Verification items for the finished model (mm, model axes). Face numbers are marked on the shaded views. Round coordinates to 2 decimals unless told otherwise and drop trailing zeros. Order: outer loops, then holes, each group sorted by start corner. A loop starts at its lowest first (then second) coordinate and runs counter-clockwise, first axis right, second up. Notation, with made-up numbers: M 47.25,3.25 L 65.25,3.25 A19 cw 65.25,17.25 Z; hole C 67,89.25 d5. An arc over 180 degrees is marked long. Use CSV: the item, a comma, the result in double quotes. Start each with the question number.
Q1. Scan lines: line 1 (Y direction, x = -77, z = 3.75) (1 decimal); line 2 (X direction, y = 24, z = 4.25); line 3 (Z direction, x = -8, y = -4). Record each from-to range of solid material in increasing order.
Q2. Sectioned sample at A-A (z = 2.75). Enter the section's corners in (x, y), and give its area (3 significant figures).
Q3. Sectioned sample at D-D (x = -106). Enter the section's corners in (y, z), and give its area (3 significant figures).
Q4. Gauge pin test, flat ends, axial feed: pin 1 Ø5 at (x, y) = (-81.5, -31.5) entering from -Z; pin 2 Ø6.5 at (x, y) = (80, 26) entering from -Z; pin 3 Ø1 at (y, z) = (25, 0) entering from -X; pin 4 Ø1.7 at (y, z) = (-24, -2) entering from -X. Record the tip position at first contact, or that the pin passes through.
Q5. Sectioned sample at B-B (y = -12.5). Enter the section's corners in (x, z).
Q6. Sectioned sample at C-C (x = 53). Enter the section's corners in (y, z).
Q7. Mould release check, pull along X, two halves, no side actions. Record for the marked faces 1, 2, 3 and 4: +X half, -X half, draft (parallel to the pull), parting line (faces both ways), or undercut.
```python
from build123d import *

# Parameters (mm, degrees)
F2_DEPTH  = 3
F3_DEPTH  = 7.9
F4_DEPTH  = 7.9
F5_DEPTH  = 3
F6_R      = 5
F6_2_R    = 5
F9_D      = 3
F10_DEPTH = 4
F11_DEPTH = 4


with BuildPart() as f2:
    # F0 (on Top) → F2 (new body)
    with BuildSketch(Plane.XY):
        with BuildLine():
            ThreePointArc((68.6448413014, 3.4252903424), (74.3230858808, 21.4851908555), (83.8, 37.8739237785))
            Line((83.8, 37.8739237785), (-65.6162592679, 37.8739237785))
            ThreePointArc((-65.6162592679, 37.8739237785), (-82.3199649398, 11.4193737584), (-82.519158721, -19.8666825891))
            Line((-82.519158721, -19.8666825891), (-73.9695476283, -37.2867286205))
            Line((-73.9695476283, -37.2867286205), (83.8, -37.2867286205))
            ThreePointArc((83.8, -37.2867286205), (75.2631412951, -21.4263167299), (69.0877699379, -4.5060504646))
            ThreePointArc((69.0877699379, -4.5060504646), (68.3487291916, -0.5692843065), (68.6448413014, 3.4252903424))
        make_face()
    extrude(amount=-F2_DEPTH)


with BuildPart() as f3:
    # F0 (on Top) → F3 (new body)
    with BuildSketch(Plane.XY):
        with BuildLine():
            ThreePointArc((-82.519158721, -19.8666825891), (-82.3199649398, 11.4193737584), (-65.6162592679, 37.8739237785))
            Line((-65.6162592679, 37.8739237785), (-99.2088739193, 37.8739237785))
            ThreePointArc((-99.2088739193, 37.8739237785), (-117.1879721114, 26.6373104948), (-114.9666717313, 5.5523567478))
            Line((-114.9666717313, 5.5523567478), (-81.4747432756, -37.2867286205))
            Line((-81.4747432756, -37.2867286205), (-73.9695476283, -37.2867286205))
            Line((-73.9695476283, -37.2867286205), (-82.519158721, -19.8666825891))
        make_face()
    extrude(amount=F3_DEPTH)


with BuildPart() as f4:
    # F0 (on Top) → F4 (new body)
    with BuildSketch(Plane.XY):
        with BuildLine():
            Line((83.8, -37.2867286205), (83.8, 37.8739237785))
            ThreePointArc((83.8, 37.8739237785), (74.3230858808, 21.4851908555), (68.6448413014, 3.4252903424))
            ThreePointArc((68.6448413014, 3.4252903424), (68.3487291916, -0.5692843065), (69.0877699379, -4.5060504646))
            ThreePointArc((69.0877699379, -4.5060504646), (75.2631412951, -21.4263167299), (83.8, -37.2867286205))
        make_face()
    extrude(amount=F4_DEPTH)


with BuildPart() as f5:
    # F5 (new): a face of the model
    f5_faces = [f3.part.faces().sort_by_distance(p)[0] for p in [
        (-94.9777366474, 10.3847598955, 0),
    ]]
    extrude(f5_faces, amount=F5_DEPTH)

    # F6#2
    f6_2_edges = [f5.edges().sort_by_distance(p)[0] for p in [
        (-81.474743, -37.286729, -1.5),
    ]]
    fillet(f6_2_edges, radius=F6_2_R)


with BuildPart() as f5b:
    # F5#2 (new): a face of the model
    f5_2_faces = [f4.part.faces().sort_by_distance(p)[0] for p in [
        (77.989714527, 0.7740894227, 0),
    ]]
    extrude(f5_2_faces, amount=F5_DEPTH)


with BuildPart() as f3_1:
    add(f3.part)

    # F6
    f6_edges = [f3_1.edges().sort_by_distance(p)[0] for p in [
        (-81.474743, -37.286729, 3.95),
    ]]
    fillet(f6_edges, radius=F6_R)


with BuildPart() as f2_1:
    add(f2.part)

    # F7: union F3, F4, F5, F5b
    add(f3_1.part)
    add(f4.part)
    add(f5.part)
    add(f5b.part)

    # F9 (through all)
    with Locations(Plane(origin=(0, 0, -3), x_dir=(1, 0, 0), z_dir=(0, 0, -1))):
        with Locations((-81.1894536018, 31.5095931292), (-113.9387488365, -24.5540793985), (-76.3550326228, -33.2092493773), (80.1921039701, 23.663148284), (80.1921039701, -25.700064376)):
            Hole(F9_D / 2)

    # F8 (on face) → F10 (cut)
    with BuildSketch(Plane(origin=(0, 0, -3), x_dir=(1, 0, 0), z_dir=(0, 0, -1))):
        Polygon((-74.5737203647, -36.1802637897), (-72.8914025376, -33.1520949158), (-74.6727147957, -30.1810805034), (-78.136344881, -30.2382349648), (-79.8186627081, -33.2664038387), (-78.0373504499, -36.2374182511), align=None)
        Polygon((83.1921039701, 21.9310974764), (83.1921039701, 25.3951990915), (80.1921039701, 27.1272498991), (77.1921039701, 25.3951990915), (77.1921039701, 21.9310974764), (80.1921039701, 20.1990466688), align=None)
        Polygon((83.1921039701, -27.4321151836), (83.1921039701, -23.9680135684), (80.1921039701, -22.2359627609), (77.1921039701, -23.9680135684), (77.1921039701, -27.4321151836), (80.1921039701, -29.1641659911), align=None)
        Polygon((-79.8767595984, 28.3038429122), (-77.7568454741, 31.043544375), (-79.0695394775, 34.249294592), (-82.5021476052, 34.7153433461), (-84.6220617296, 31.9756418833), (-83.3093677262, 28.7698916664), align=None)
        Polygon((-110.4805015339, -24.7553890954), (-112.0352858737, -21.6598042304), (-115.4935331763, -21.4584945334), (-117.3969961391, -24.3527697016), (-115.8422117994, -27.4483545667), (-112.3839644968, -27.6496642636), align=None)
    extrude(amount=-F10_DEPTH, mode=Mode.SUBTRACT)

    # F8 (on face) → F11 (cut)
    with BuildSketch(Plane(origin=(0, 0, -3), x_dir=(1, 0, 0), z_dir=(0, 0, -1))):
        Polygon((-74.5737203647, -36.1802637897), (-72.8914025376, -33.1520949158), (-74.6727147957, -30.1810805034), (-78.136344881, -30.2382349648), (-79.8186627081, -33.2664038387), (-78.0373504499, -36.2374182511), align=None)
        Polygon((83.1921039701, 21.9310974764), (83.1921039701, 25.3951990915), (80.1921039701, 27.1272498991), (77.1921039701, 25.3951990915), (77.1921039701, 21.9310974764), (80.1921039701, 20.1990466688), align=None)
        Polygon((83.1921039701, -27.4321151836), (83.1921039701, -23.9680135684), (80.1921039701, -22.2359627609), (77.1921039701, -23.9680135684), (77.1921039701, -27.4321151836), (80.1921039701, -29.1641659911), align=None)
        Polygon((-79.8767595984, 28.3038429122), (-77.7568454741, 31.043544375), (-79.0695394775, 34.249294592), (-82.5021476052, 34.7153433461), (-84.6220617296, 31.9756418833), (-83.3093677262, 28.7698916664), align=None)
        Polygon((-110.4805015339, -24.7553890954), (-112.0352858737, -21.6598042304), (-115.4935331763, -21.4584945334), (-117.3969961391, -24.3527697016), (-115.8422117994, -27.4483545667), (-112.3839644968, -27.6496642636), align=None)
    extrude(amount=-F11_DEPTH, mode=Mode.SUBTRACT)


solid = f2_1.part
```
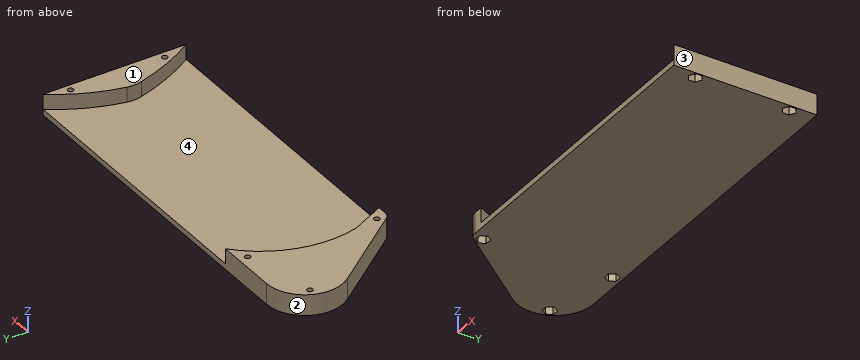
Verdict:
1,line 1,"y = -37.3 to -31.1, 23.9 to 31.9, 34.6 to 37.9"
1,line 2,"x = -118.25 to -115.33, -112.54 to -76.92, 75.48 to 83.8"
1,line 3,"z = -3 to 0"
2,outline,"M -114.97,5.55 L -82.98,-35.37 A5 ccw -79.04,-37.29 L -73.97,-37.29 L -82.52,-19.87 A56.92 cw -65.62,37.87 L -99.21,37.87 A20 ccw Z; M 68.64,3.43 A15.48 ccw 69.09,-4.51 A125.34 ccw 83.8,-37.29 L 83.8,37.87 A86.36 ccw Z; hole C -113.94,24.55 d3; hole C -81.19,-31.51 d3; hole C -76.36,33.21 d3; hole C 80.19,-23.66 d3; hole C 80.19,25.7 d3"
2,area,"2,640 mm²"
3,outline,"M -5.92,-3 L 36.69,-3 L 36.69,7.9 L -5.92,7.9 Z"
3,area,"464 mm²"
4,pin 1,"stops at z = 1"
4,pin 2,"stops at z = -3"
4,pin 3,"stops at x = -118.08"
4,pin 4,"stops at x = -92.53"
5,outline,"M -100.85,-3 L 83.8,-3 L 83.8,7.9 L 71.66,7.9 L 71.66,0 L -84.06,0 L -84.06,7.9 L -100.85,7.9 Z"
6,outline,"M -37.29,-3 L 37.87,-3 L 37.87,0 L -37.29,0 Z"
7,face 1,"draft"
7,face 2,"-X half"
7,face 3,"+X half"
7,face 4,"undercut"
